```python
from build123d import *

# Parameters (mm, degrees)
SKETCH1_W           = 54.61
SKETCH1_H           = 55.88
BOSS_EXTRUDE1_DEPTH = 1.6
SKETCH2_R           = 1.59938652
SKETCH2_R_2         = 1.593077756
SKETCH2_R_3         = 0.452574799
SKETCH2_R_4         = 0.480028064
SKETCH2_R_5         = 0.465129332
SKETCH2_R_6         = 0.486649453
SKETCH2_R_7         = 1.565869332
SKETCH2_R_8         = 0.397895911
SKETCH2_R_9         = 0.397882454
SKETCH2_R_10        = 0.356595037
SKETCH2_R_11        = 0.333594003
SKETCH2_R_12        = 0.239542347
SKETCH2_R_13        = 0.226201547
SKETCH2_R_14        = 0.233275918
SKETCH2_R_15        = 0.256166525
SKETCH2_R_16        = 0.255392926
SKETCH2_R_17        = 0.248136055
SKETCH2_R_18        = 0.447662922
SKETCH2_R_19        = 0.452252407
SKETCH2_R_20        = 0.239942714
SKETCH2_R_21        = 0.391464076
SKETCH2_R_22        = 0.360331554
SKETCH2_R_23        = 0.404490663
SKETCH2_R_24        = 0.384788584
SKETCH2_R_25        = 0.257107561
SKETCH2_R_26        = 0.273253907
SKETCH2_R_27        = 0.39651489
SKETCH2_R_28        = 0.393350562
SKETCH2_R_29        = 0.355618877
SKETCH2_R_30        = 0.377526949
SKETCH2_R_31        = 0.377766955
SKETCH2_R_32        = 0.36325523
SKETCH2_R_33        = 0.378551554
SKETCH2_R_34        = 0.355329697
SKETCH2_R_35        = 0.382997324
SKETCH2_R_36        = 0.369709734
SKETCH2_R_37        = 0.37124433
SKETCH2_R_38        = 0.385916857
SKETCH2_R_39        = 0.363938308
SKETCH2_R_40        = 0.333537697
SKETCH2_R_41        = 0.310028392
SKETCH2_R_42        = 0.333886041
SKETCH2_R_43        = 0.330283809
SKETCH2_R_44        = 0.364374395
SKETCH2_R_45        = 0.353792472
SKETCH2_R_46        = 0.372885559
SKETCH2_R_47        = 0.348600153
SKETCH2_R_48        = 0.384803628
SKETCH2_R_49        = 0.387591086
SKETCH2_R_50        = 0.354490901
SKETCH2_R_51        = 0.415876944
SKETCH2_R_52        = 0.351498041
SKETCH2_R_53        = 0.392374017
SKETCH2_R_54        = 0.434288257
SKETCH2_R_55        = 0.292605843
SKETCH2_R_56        = 0.335537626
SKETCH2_R_57        = 1.564224328
SKETCH2_R_58        = 0.508580285
SKETCH2_R_59        = 0.555593041
SKETCH2_R_60        = 0.530092741
SKETCH2_R_61        = 0.459629548
SKETCH2_R_62        = 0.465333024
CUT_EXTRUDE1_DEPTH  = 2.6


with BuildPart() as part:
    # Sketch1 → Boss-Extrude1 (new body)
    with BuildSketch(Plane(origin=(0, 0, 0), x_dir=(1, 0, 0), z_dir=(0, 1, 0))):
        Rectangle(SKETCH1_W, SKETCH1_H)
    extrude(amount=BOSS_EXTRUDE1_DEPTH)

    # Sketch2 → Cut-Extrude1 (cut, through all)
    with BuildSketch(Plane(origin=(0, 1.6, 0), x_dir=(1, 0, 0), z_dir=(0, 1, 0))):
        with Locations((-16.664297308, 23.932043145)):
            Circle(SKETCH2_R)
        with Locations((10.980265243, 14.950869261)):
            Circle(SKETCH2_R_2)
        with Locations((16.166703819, 17.6326375)):
            Circle(SKETCH2_R_3)
        with Locations((16.166703819, 22.060085065)):
            Circle(SKETCH2_R_4)
        with Locations((22.567528012, 22.060085065)):
            Circle(SKETCH2_R_5)
        with Locations((22.567528012, 17.6326375)):
            Circle(SKETCH2_R_6)
        with Locations((-8.213065376, -1.3990828)):
            Circle(SKETCH2_R_7)
        with Locations((-12.880776497, -0.068306864)):
            Circle(SKETCH2_R_8)
        with Locations((-15.367822181, -0.068306864)):
            Circle(SKETCH2_R_9)
        with Locations((-17.854706203, -0.068306864)):
            Circle(SKETCH2_R_10)
        with Locations((-20.312369623, -0.068306864)):
            Circle(SKETCH2_R_11)
        with Locations((-20.075921844, -5.738541726)):
            Circle(SKETCH2_R_12)
        with Locations((-15.704587313, -10.428115561)):
            Circle(SKETCH2_R_13)
        with Locations((-11.307135458, -12.45851306)):
            Circle(SKETCH2_R_14)
        with Locations((-13.190051269, -13.04767065)):
            Circle(SKETCH2_R_15)
        with Locations((-15.784379921, -12.883809097)):
            Circle(SKETCH2_R_16)
        with Locations((-22.431122431, -12.765558111)):
            Circle(SKETCH2_R_17)
        with Locations((-25.275605658, -10.917044443)):
            Circle(SKETCH2_R_18)
        with Locations((-25.275605658, -3.991987316)):
            Circle(SKETCH2_R_19)
        with Locations((-16.705936806, -16.421463043)):
            Circle(SKETCH2_R_20)
        with Locations((-12.880776497, -17.459342868)):
            Circle(SKETCH2_R_21)
        with Locations((-12.880776497, -22.375845154)):
            Circle(SKETCH2_R_22)
        with Locations((-2.983360407, -22.375845154)):
            Circle(SKETCH2_R_23)
        with Locations((-2.983360407, -17.459342868)):
            Circle(SKETCH2_R_24)
        with Locations((3.427815902, -17.319364157)):
            Circle(SKETCH2_R_25)
        with Locations((-7.932777582, -11.644816009)):
            Circle(SKETCH2_R_26)
        with Locations((-2.983360407, -9.935549628)):
            Circle(SKETCH2_R_27)
        with Locations((-2.983360407, -7.480563575)):
            Circle(SKETCH2_R_28)
        with Locations((-2.983360407, -4.987813874)):
            Circle(SKETCH2_R_29)
        with Locations((-2.983360407, -2.521390191)):
            Circle(SKETCH2_R_30)
        with Locations((-2.983360407, -0.068306864)):
            Circle(SKETCH2_R_31)
        with Locations((-2.983360407, 2.444706456)):
            Circle(SKETCH2_R_32)
        with Locations((-2.983360407, 4.893099371)):
            Circle(SKETCH2_R_33)
        with Locations((-2.983360407, 7.385639552)):
            Circle(SKETCH2_R_34)
        with Locations((-2.983360407, 9.849195982)):
            Circle(SKETCH2_R_35)
        with Locations((-2.983360407, 12.363056337)):
            Circle(SKETCH2_R_36)
        with Locations((-2.983360407, 14.833883975)):
            Circle(SKETCH2_R_37)
        with Locations((-2.983360407, 17.348014362)):
            Circle(SKETCH2_R_38)
        with Locations((-2.983360407, 19.737222803)):
            Circle(SKETCH2_R_39)
        with Locations((-2.983360407, 22.277194941)):
            Circle(SKETCH2_R_40)
        with Locations((4.456862321, 19.737222803)):
            Circle(SKETCH2_R_41)
        with Locations((4.456862321, 22.277194941)):
            Circle(SKETCH2_R_42)
        with Locations((4.456862321, 17.348014362)):
            Circle(SKETCH2_R_43)
        with Locations((4.456862321, 14.833883975)):
            Circle(SKETCH2_R_44)
        with Locations((4.456862321, 12.363056337)):
            Circle(SKETCH2_R_45)
        with Locations((4.456862321, 9.849195982)):
            Circle(SKETCH2_R_46)
        with Locations((4.456862321, 7.385639552)):
            Circle(SKETCH2_R_47)
        with Locations((4.456862321, 4.893099371)):
            Circle(SKETCH2_R_48)
        with Locations((4.456862321, 2.444706456)):
            Circle(SKETCH2_R_49)
        with Locations((4.456862321, -0.068306864)):
            Circle(SKETCH2_R_50)
        with Locations((4.456862321, -2.521390191)):
            Circle(SKETCH2_R_51)
        with Locations((4.456862321, -4.987813874)):
            Circle(SKETCH2_R_52)
        with Locations((4.456862321, -7.480563575)):
            Circle(SKETCH2_R_53)
        with Locations((4.456862321, -9.935549628)):
            Circle(SKETCH2_R_54)
        with Locations((10.669719496, -1.304797587)):
            Circle(SKETCH2_R_55)
        with Locations((10.669719496, 3.682313247)):
            Circle(SKETCH2_R_56)
        with Locations((10.377113652, -13.101088656)):
            Circle(SKETCH2_R_57)
        with Locations((20.92912061, -16.421463043)):
            Circle(SKETCH2_R_58)
        with Locations((20.92912061, -20.789810067)):
            Circle(SKETCH2_R_59)
        with Locations((24.309641026, 1.206553039)):
            Circle(SKETCH2_R_60)
        with Locations((24.309641026, -1.304797587)):
            Circle(SKETCH2_R_61)
        with Locations((24.309641026, -3.770776983)):
            Circle(SKETCH2_R_62)
    extrude(amount=-CUT_EXTRUDE1_DEPTH, mode=Mode.SUBTRACT)


solid = part.part
```
Geometry: final body of the model. Coordinates: model frame, mm. Round coordinates to 2 decimals unless told otherwise and drop trailing zeros. Use one line per item in the form item = value. Start each with the question number.
1) Line query: L1, parallel to X at y = 0.4, z = -7.5 (3 decimals); L2, parallel to X at y = 0.9, z = 10 (3 decimals); L3, parallel to X at y = 1.1, z = -15 (3 decimals). Output: solid intervals per line, ascending.
2) Section A-A on y = 0.4. Give the number of separate pieces and of enclosed holes in the cut face, then the cut area to 3 significant figures.
3) First-contact query: P1, Ø0.9, axis at x = 20.93, z = 20.79, coming from the -Y side. Flat tip, straight axial feed; report the tip coordinate or a pass-through.
4) Draft query along X for faces 1 (the cylindrical face through (9.136, 0.811, 14.053)), 2 (the flat face through (-27.305, 1, 0)), 3 (the flat face through (27.305, 1, 0)), 4 (the flat face through (0, 0, 0)). Return one class per face: released by +X, released by -X, zero draft, split by the parting line, or undercut.
Response:
q1.L1 = -27.305 to -3.32, -2.647 to 4.128, 4.786 to 27.305
q1.L2 = -27.305 to -3.375, -2.592 to 4.027, 4.886 to 27.305
q1.L3 = -27.305 to -3.315, -2.651 to 4.133, 4.781 to 9.388, 12.573 to 27.305
q2.separate_pieces = 1
q2.enclosed_holes = 62
q2.area = 2,990 mm^2
q3.P1 = through
q4.face_1 = undercut
q4.face_2 = released by -X
q4.face_3 = released by +X
q4.face_4 = zero draft
